Geometry check sheet. Reference: the model listing, model coordinates, mm. Face numbers are marked on the shaded views. A direction names the side the tool comes from. Round coordinates to 2 decimals unless told otherwise and drop trailing zeros. Order: outer loops, then holes, each group sorted by start corner. A loop starts at its lowest first (then second) coordinate and runs counter-clockwise, first axis right, second up. Notation, with made-up numbers: (56.5, -25) - (76.5, -25) arc R14 cw to (76.5, -20) - close; hole circle Ø7 at (64, -10.75). An arc over 180 degrees is marked (long way). Return JSON: item names as keys, results as strings. Group by question number.
Q1. Gauge pin test, flat ends, axial feed: pin 1 Ø0.6 at (x, y) = (17, 5.5) entering from -Z; pin 2 Ø2.5 at (x, y) = (0, 6) entering from +Z; pin 3 Ø1 at (y, z) = (5, 3) entering from +X; pin 4 Ø1.5 at (y, z) = (3.5, -13) entering from -X. Record the tip position at first contact, or that the pin passes through.
Q2. Sectioned sample at A-A, the plane z = 0. Give the number of separate pieces and of enclosed holes in the cut face, then the cut area to 3 significant figures.
Q3. Sectioned sample at D-D, the plane y = 0.5. Record the cut outline in (x, z).
Q4. Material ranges on line 1 along Y through (x, z) = (19.15, 0); line 2 along Z through (x, y) = (0, 2.1); line 3 along X through (y, z) = (6, -14.75), recorded low to high.
Q5. Tool access check on the marked faces 1, 2, 3, 4 and 5. Record the directions out of +Z, -Z, +X, -X, +Y, -Y that give a thin tool (end or side, any length) a straight path to the whole face; none if there is none.
Q6. Sectioned sample at C-C, the plane x = 11.5. Record the cut outline in (y, z).
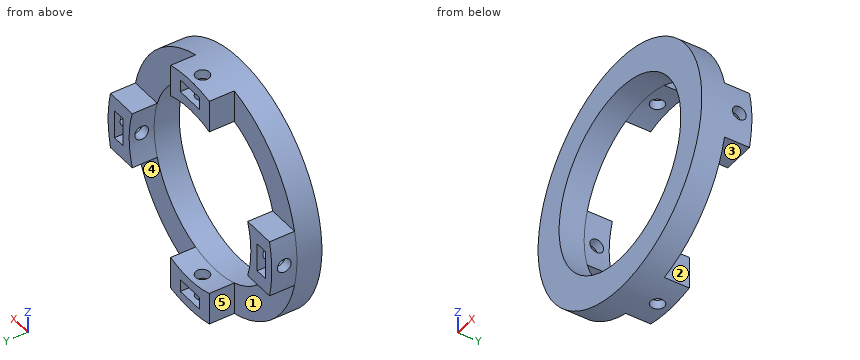
```python
from build123d import *
from build123d.topology import SkipClean

# Parameters (mm, degrees)
SKETCH_1_R               = 19.5
SKETCH_1_R_2             = 14.5
EXTRUDE_1_DEPTH          = 4
SKETCH_3_W               = 4.6
SKETCH_3_H               = 2
SKETCH_3_W_2             = 2
SKETCH_3_H_2             = 4.6
EXTRUDE_3_DEPTH          = 4
SKETCH_12_R              = 1.1
CUT_EXTRUDE_2_DEPTH      = 44.017438324
PATTERN_CIRCULAR_2_COUNT = 2
PATTERN_CIRCULAR_2_ANGLE = 90


with BuildPart() as part:
    # Эскиз1 → Бобышка-Вытянуть1 (new body)
    with BuildSketch(Plane(origin=(0, 0, 0), x_dir=(1, 0, 0), z_dir=(0, 1, 0))):
        with Locations(Location((0, 0, 0), (0, 0, 270))):
            Circle(SKETCH_1_R)
        with Locations(Location((0, 0, 0), (0, 0, 270))):
            Circle(SKETCH_1_R_2, mode=Mode.SUBTRACT)
    extrude(amount=EXTRUDE_1_DEPTH)

    # Эскиз3 → Бобышка-Вытянуть3 (add)
    # profile 1 of 4: a face of its own
    with SkipClean():  # the faces are left unmerged after this step: merging them gives an invalid solid
        with BuildSketch(Plane(origin=(0, 4, 0), x_dir=(1, 0, 0), z_dir=(0, 1, 0))):
            with BuildLine():
                Line((-4.599991072, 18.949672349), (-4.599991072, 13.75100295))
                ThreePointArc((-4.599991072, 13.75100295), (0, 14.5), (4.599991072, 13.75100295))
                Line((4.599991072, 13.75100295), (4.599991072, 18.949672349))
                ThreePointArc((4.599991072, 18.949672349), (0, 19.5), (-4.599991072, 18.949672349))
            make_face()
            with Locations((0, 17)):
                Rectangle(SKETCH_3_W, SKETCH_3_H, mode=Mode.SUBTRACT)
        # profile 2 of 4: a face of its own
        with BuildSketch(Plane(origin=(0, 4, 0), x_dir=(1, 0, 0), z_dir=(0, 1, 0))):
            with BuildLine():
                Line((18.949672349, 4.599991072), (13.75100295, 4.599991072))
                ThreePointArc((13.75100295, 4.599991072), (14.5, 0), (13.75100295, -4.599991072))
                Line((13.75100295, -4.599991072), (18.949672349, -4.599991072))
                ThreePointArc((18.949672349, -4.599991072), (19.5, 0), (18.949672349, 4.599991072))
            make_face()
            with Locations((17, 0)):
                Rectangle(SKETCH_3_W_2, SKETCH_3_H_2, mode=Mode.SUBTRACT)
        # profile 3 of 4: a face of its own
        with BuildSketch(Plane(origin=(0, 4, 0), x_dir=(1, 0, 0), z_dir=(0, 1, 0))):
            with BuildLine():
                Line((4.599991072, -18.949672349), (4.599991072, -13.75100295))
                ThreePointArc((4.599991072, -13.75100295), (0, -14.5), (-4.599991072, -13.75100295))
                Line((-4.599991072, -13.75100295), (-4.599991072, -18.949672349))
                ThreePointArc((-4.599991072, -18.949672349), (0, -19.5), (4.599991072, -18.949672349))
            make_face()
            with Locations((0, -17)):
                Rectangle(SKETCH_3_W, SKETCH_3_H, mode=Mode.SUBTRACT)
        # profile 4 of 4: a face of its own
        with BuildSketch(Plane(origin=(0, 4, 0), x_dir=(1, 0, 0), z_dir=(0, 1, 0))):
            with BuildLine():
                Line((-18.949672349, -4.599991072), (-13.75100295, -4.599991072))
                ThreePointArc((-13.75100295, -4.599991072), (-14.5, 0), (-13.75100295, 4.599991072))
                Line((-13.75100295, 4.599991072), (-18.949672349, 4.599991072))
                ThreePointArc((-18.949672349, 4.599991072), (-19.5, 0), (-18.949672349, -4.599991072))
            make_face()
            with Locations((-17, 0)):
                Rectangle(SKETCH_3_W_2, SKETCH_3_H_2, mode=Mode.SUBTRACT)
        extrude(amount=EXTRUDE_3_DEPTH)

    # Эскиз12 → Вырез-Вытянуть2 (cut, symmetric)
    with SkipClean():  # the faces are left unmerged after this step: merging them gives an invalid solid
        with BuildSketch(Plane.XY.offset(-18)):
            with Locations((0, 6)):
                Circle(SKETCH_12_R)
        cut_extrude_2 = extrude(amount=CUT_EXTRUDE_2_DEPTH, both=True, mode=Mode.SUBTRACT)

    # Круговой массив2: Вырез-Вытянуть2 ×2 about axis
    with SkipClean():  # the faces are left unmerged after this step: merging them gives an invalid solid
        pattern_circular_2_axis = Axis((0, 4, 0), (0, -1, 0))
        for i in range(1, PATTERN_CIRCULAR_2_COUNT):
            add(cut_extrude_2.rotate(pattern_circular_2_axis, i * PATTERN_CIRCULAR_2_ANGLE / (PATTERN_CIRCULAR_2_COUNT - 1)), mode=Mode.SUBTRACT)


solid = part.part
```
Reply:
{
 "1": {"pin 1": "z = -4.6", "pin 2": "z = 19.5", "pin 3": "x = 19.34", "pin 4": "x = -15.17"},
 "2": {"separate pieces": "6", "enclosed holes": "0", "area": "50.8 mm^2"},
 "3": {"outline": "circle Ø39 at (0, 0); hole circle Ø29 at (0, 0)"},
 "4": {"line 1": "0 to 4.9, 7.1 to 8", "line 2": "-19.5 to -14.5, 14.5 to 19.5", "line 3": "-4.6 to -1.1, 1.1 to 4.6"},
 "5": {"face 1": "-Z, -X, +Y", "face 2": "+Z, -Z, +X, +Y", "face 3": "-Z, +X, -X, +Y", "face 4": "-Z, +X, +Y", "face 5": "+Z, -Z, -X, +Y"},
 "6": {"outline": "(0, -15.75) - (4, -15.75) - (4, -8.83) - (0, -8.83) - close; (0, 8.83) - (4, 8.83) - (4, 15.75) - (0, 15.75) - close"}
}
